Geometry: final body of the model. Coordinates: model frame, mm. A direction names the side the tool comes from. Give positions to 0.01 mm unless a question says otherwise; leave off trailing zeros. Write each loop counter-clockwise with the first axis right and the second up, starting at its lowest first coordinate (ties: lowest second). Pieces come first, ordered by that corner, then holes. Notation, with made-up numbers: (16, 64) -> (50, 64) arc R9 ccw to (50, 77) -> close; hole circle Ø8 at (77.5, 54). An arc over 180 degrees is marked (long way). Answer as a JSON object with one key per item and string values. Group by question number.
(1) Draft query along Y for faces 3 (the face through (-18, 6, 29)), 4 (the face through (0, 0, 29)), 5 (the face through (18, 4, 55)), 6 (the face through (-19, 3, 29)). Return one class per face: +Y half, -Y half, draft (parallel to the pull), parting line (faces both ways), or undercut.
(2) Section query A-A on z = 2. Output: boundary loops of the cut face in (x, y).
(3) Material intervals for probe 1 along X at (y, z) = (4, 4); probe 2 along Y at (x, z) = (17.85, 54); probe 3 along Y at (x, z) = (-6, 12.5), sorted ascending.
(4) Section query C-C on x = -13. Output: boundary loops of the cut face in (y, z).
(5) Contact query for a flat-ended pin moving along its axis: pin 1 Ø10 at (x, z) = (-3.5, 17) entering from +Y. Output: stop coordinate, or through.
(6) Set-up query: faces 1 (the face through (17, 4, 29)), 2 (the face through (18, 5, 2)). Return all of +Z, -Z, +X, -X, +Y, -Y with unobstructed straight access to the full face (end or side cutting, diameter ignored); none if empty.
(7) Section query B-B on z = 29. Output: boundary loops of the cut face in (x, y).
Autodesk Inventor part; units mm, degrees
ref_plane "YZ Plane" through (0, 0, 0) normal (1, 0, 0) x (0, 1, 0)
ref_plane "XZ Plane" through (0, 0, 0) normal (0, 1, 0) x (-1, 0, 0)
ref_plane "XY Plane" through (0, 0, 0) normal (0, 0, 1) x (1, 0, 0)
sketch "草图1" plane through (0, 0, 0) normal (0, 0, 1) x (1, 0, 0)
  line L0 (0, -1.2) -> (0, 7.2) construction
  line L1 (-26.6, 0) -> (26.6, 0) construction
  line L2 (0, 0) -> (-19, 0)
  line L3 (0, 2) -> (-17, 2)
  line L4 (-19, 0) -> (-19, 6)
  line L5 (-19, 6) -> (-17, 6)
  line L6 (-17, 6) -> (-17, 2)
  line L7 (0, 0) -> (19, 0)
  line L8 (0, 2) -> (17, 2)
  line L9 (19, 0) -> (19, 6)
  line L10 (19, 6) -> (17, 6)
  line L11 (17, 6) -> (17, 2)
  dimension "d0" = 19
  dimension "d1" = 17
  dimension "d2" = 2
  dimension "d3" = 6
extrude "拉伸1" add sketch "草图1" along normal blind 58
sketch "草图2" plane through (19, 0, 0) normal (1, 0, 0) x (0, 0, -1)
  line L0 (0, 6) -> (0, 0) construction
  line L1 (0, 6) -> (-58, 6) construction
  line L2 (-58, 0) -> (-58, 6) construction
  line L3 (0, 0) -> (-58, 0) construction
  line L4 (0, 2) -> (-58, 2) construction
  line L5 (0, 6) -> (-58, 6) construction
  line L6 (-56, 6) -> (-56, 0) construction
  line L7 (0, 0) -> (-58, 0) construction
  line L8 (-58, 0) -> (-58, 6) construction
  line L9 (-58, 4) -> (0, 4) construction
  circle A0 centre (-54, 4) radius 1
  circle A1 centre (-2, 4) radius 1
  dimension "d6" = 2
  dimension "d7" = 4
  dimension "d8" = 2
  dimension "d9" = 2
  dimension "d10" = 2
  dimension "d11" = 2
extrude "拉伸2" cut sketch "草图2" against normal blind 2
mirror "镜像1" about plane through (0, 0, 0) normal (1, 0, 0) of "拉伸2"
properties part number "CaseBottom"
Answer list:
{
 "1": {"face 3": "+Y half", "face 4": "-Y half", "face 5": "undercut", "face 6": "draft"},
 "2": {"outline": "(-19, 0) -> (19, 0) -> (19, 3) -> (17, 3) -> (17, 2) -> (-17, 2) -> (-17, 3) -> (-19, 3) -> close; (-19, 5) -> (-17, 5) -> (-17, 6) -> (-19, 6) -> close; (17, 5) -> (19, 5) -> (19, 6) -> (17, 6) -> close"},
 "3": {"probe 1": "-19 to -17, 17 to 19", "probe 2": "0 to 3, 5 to 6", "probe 3": "0 to 2"},
 "4": {"outline": "(0, 0) -> (2, 0) -> (2, 58) -> (0, 58) -> close"},
 "5": {"pin 1": "y = 2"},
 "6": {"face 1": "+Z, -Z, +Y", "face 2": "+X, -X"},
 "7": {"outline": "(-19, 0) -> (19, 0) -> (19, 6) -> (17, 6) -> (17, 2) -> (-17, 2) -> (-17, 6) -> (-19, 6) -> close"}
}
